Could you check a few things on this model? Use its own coordinates, in mm. A direction names the side the tool comes from. Give positions to 0.01 mm unless a question says otherwise; leave off trailing zeros. Loops run counter-clockwise (first coordinate to the right, second up) from the corner with the lowest first, then second, coordinate; pieces in that order, holes last. Notation, with made-up numbers: (47, 41) -> (53, 41) arc R16 cw to (53, 65) -> close; hole circle Ø2 at (39, 47). An arc over 180 degrees is marked (long way). Write each question's results on one line, items separated by ' | '. Start each with the question number.
Q1. If we section it at A-A, the plane x = 74: List the corners of the cut face in (y, z) for me (3 decimals), plus the area to 3 significant figures.
Q2. We'd pull the mould along X, two halves only. Please class faces 5 (the face through (11, 12, -0.8)), 6 (the face through (52, 9, 3)), 7 (the face through (65.459, -8.827, 4.762)): released by +X, released by -X, zero draft, split by the parting line, or undercut.
Q3. If I drill on line 1 along X through (y, z) = (9.5, 3.5); line 2 along X through (y, z) = (9, 5.5); line 3 along Y through (x, z) = (5.5, 4.25), over which ranges is the centre line in solid material (lowest first)?
Q4. Will these pins go through, and if not, where does the flat tip stop? P1, Ø2.5, axis at x = 92.5, y = -21, coming from the -Z side; P2, Ø2.5, axis at x = 90.34, y = 8.33, coming from the -Z side; P3, Ø3.5, axis at x = 4, z = 4.5, coming from the -Y side; P4, Ø1.1, axis at y = 7.5, z = 5, coming from the +X side.
Q5. If we section it at B-B, the plane z = 1.75: List the corners of the cut face in (x, y) for me (3 decimals).
Q6. If we section it at C-C, the plane y = -13.5: List the corners of the cut face in (x, z) for me (3 decimals).
Q7. Which directions (+Z, -Z, +X, -X, +Y, -Y) give clear straight access to the entire face, cutting with the end or side of a thin tool? Please do faces 1 (the face through (15, 8, 5)), 2 (the face through (86.6, -22.7, 1.5)), 3 (the face through (5, 8, 0)), 4 (the face through (92.1, 6.6, 0)).
from build123d import *

# Parameters (mm, degrees)
SKETCH2_R           = 2.025
BOSS_EXTRUDE1_DEPTH = 6.575
SKETCH3_W           = 85
SKETCH3_H           = 45
SKETCH3_R           = 4
CUT_EXTRUDE1_DEPTH  = 3
BOSS_EXTRUDE2_DEPTH = 0.8


with BuildPart() as part:
    # Sketch2 → Boss-Extrude1 (new body)
    with BuildSketch(Plane.XY):
        with BuildLine():
            Line((0, 19), (0, 0))
            Line((0, 0), (13, 0))
            Line((13, 0), (89.060496565, -25.00806589))
            ThreePointArc((89.060496565, -25.00806589), (94.109744025, -22.45755612), (91.559234256, -17.40830866))
            Line((91.559234256, -17.40830866), (38.617230635, -0.001413167))
            ThreePointArc((38.617230635, -0.001413167), (35.662685114, 5.091263251), (40.379460771, 8.614999867))
            Line((40.379460771, 8.614999867), (89.992289035, 4.346816993))
            ThreePointArc((89.992289035, 4.346816993), (94.32042132, 7.989243509), (90.677994805, 12.317375794))
            Line((90.677994805, 12.317375794), (13, 19))
            Line((13, 19), (0, 19))
        make_face()
        with Locations((90.33514192, 8.332096393)):
            Circle(SKETCH2_R, mode=Mode.SUBTRACT)
        with Locations((90.30986541, -21.208187275)):
            Circle(SKETCH2_R, mode=Mode.SUBTRACT)
        with BuildLine():
            Line((15, 10.45427111), (15, 6.44857097))
            ThreePointArc((15, 6.44857097), (15.759824435, 4.103093981), (17.750631155, 2.648692356))
            Line((17.750631155, 2.648692356), (24.997412202, 0.266010331))
            ThreePointArc((24.997412202, 0.266010331), (28.242503446, 0.599321176), (30.16022559, 3.238270793))
            Line((30.16022559, 3.238270793), (31.357615095, 8.900202452))
            ThreePointArc((31.357615095, 8.900202452), (30.656648203, 12.111093006), (27.787023436, 13.713100006))
            Line((27.787023436, 13.713100006), (19.342852885, 14.43955051))
            ThreePointArc((19.342852885, 14.43955051), (16.29550481, 13.401423255), (15, 10.45427111))
        make_face(mode=Mode.SUBTRACT)
    extrude(amount=BOSS_EXTRUDE1_DEPTH)

    # Sketch3 → Cut-Extrude1 (cut)
    with BuildSketch(Plane(origin=(0, 0, 0), x_dir=(-1, 0, 0), z_dir=(0, 0, -1))):
        with Locations((-55.5, -3.5)):
            Rectangle(SKETCH3_W, SKETCH3_H)
        with Locations((-90.3351, 8.3321)):
            Circle(SKETCH3_R, mode=Mode.SUBTRACT)
        with Locations((-90.3096, -21.2081)):
            Circle(SKETCH3_R, mode=Mode.SUBTRACT)
    extrude(amount=-CUT_EXTRUDE1_DEPTH, mode=Mode.SUBTRACT)

    # Sketch4 → Boss-Extrude2 (add)
    with BuildSketch(Plane(origin=(0, 0, 0), x_dir=(-1, 0, 0), z_dir=(0, 0, -1))):
        Polygon((0, 19), (-13, 19), (-13, 0), (-10.5, 0), (-10.5, 16.5), (0, 16.5), align=None)
    extrude(amount=BOSS_EXTRUDE2_DEPTH)


solid = part.part
Final values:
1) outline: (-20.056, 3) -> (-11.635, 3) -> (-11.635, 6.575) -> (-20.056, 6.575) -> close; (5.723, 3) -> (13.752, 3) -> (13.752, 6.575) -> (5.723, 6.575) -> close | area: 58.8 mm²
2) face 5: zero draft | face 6: undercut | face 7: released by +X
3) line 1: x = 0 to 15, 31.44 to 88.68, 91.99 to 94.16 | line 2: x = 0 to 15, 31.38 to 88.42, 92.25 to 94.28 | line 3: y = 0 to 19
4) P1: stops at z = 0 | P2: passes through | P3: stops at y = 0 | P4: stops at x = 94.33
5) outline: (0, 0) -> (13, 0) -> (13, 19) -> (0, 19) -> close; circle Ø8 at (90.31, -21.208); circle Ø8 at (90.335, 8.332); hole circle Ø4.05 at (90.31, -21.208); hole circle Ø4.05 at (90.335, 8.332)
6) outline: (54.059, 3) -> (79.672, 3) -> (79.672, 6.575) -> (54.059, 6.575) -> close
7) face 1: +Z, -Z | face 2: -Z | face 3: -Z, -X, -Y | face 4: -Z, +X, +Y, -Y
